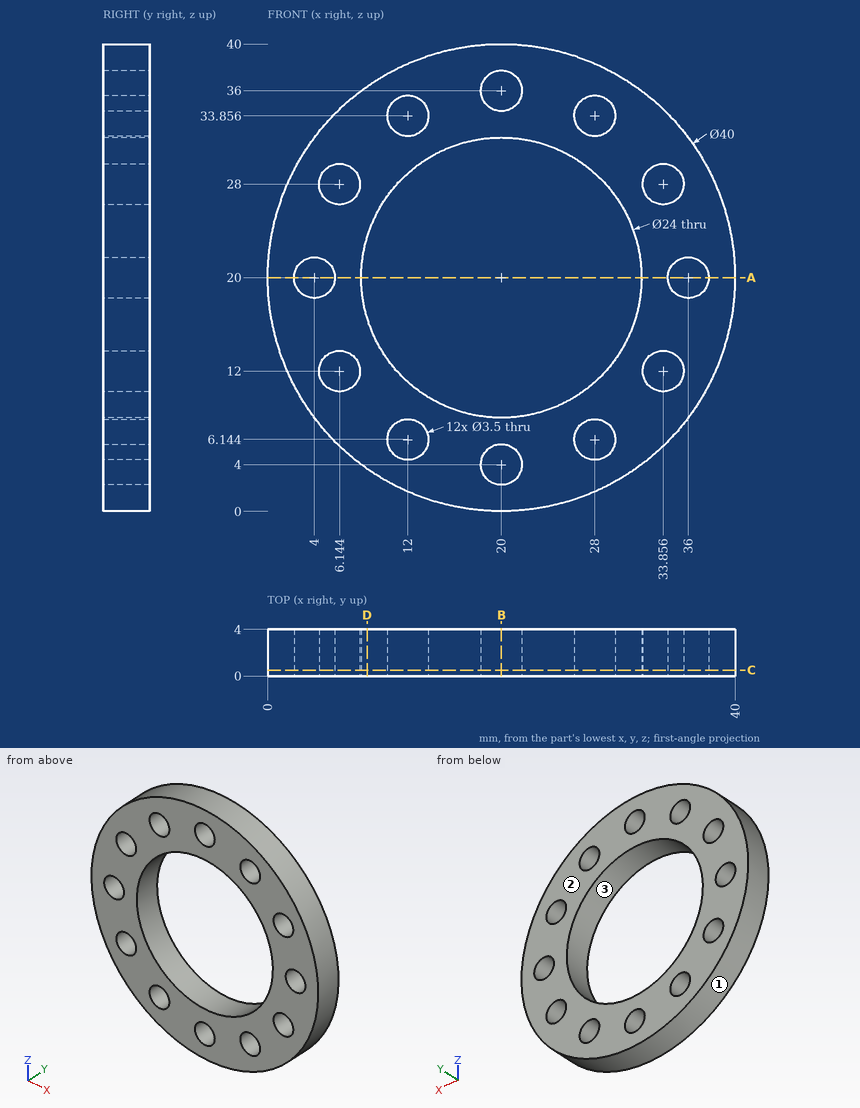
Source: three-view drawing plus pictorial views. Frame: mm from the lowest corner of the part. Give positions to 0.01 mm unless a question says otherwise; leave off trailing zeros. Write each loop counter-clockwise with the first axis right and the second up, starting at its lowest first coordinate (ties: lowest second). Pieces come first, ordered by that corner, then holes. Notation, with made-up numbers: (80, 40) - (90, 40) arc R29 ccw to (90, 74) - close; hole circle Ø7 at (49.5, 81). An arc over 180 degrees is marked (long way). Write item = value, one per line. Start each with the question number.
1. Section query A-A, the plane z = 20. Output: boundary loops of the cut face in (x, y), then the cut area to 3 significant figures.
2. Ray query, L1, parallel to X at y = 2.3, z = 20; L2, parallel to X at y = 0.8, z = 6 (1 decimal); L3, parallel to X at y = 2.95, z = 28 (1 decimal). Return the intervals inside material, ascending.
3. First-contact query: pin 1 Ø1 at (x, y) = (6, 2) entering from -Z (1 decimal); pin 2 Ø4.5 at (x, z) = (12, 6.14) entering from -Y; pin 3 Ø1 at (y, z) = (2.5, 23) entering from +X; pin 4 Ø1.5 at (x, y) = (22.5, 2) entering from -Z. Flat tips, straight axial feed; report the tip coordinate or a pass-through.
4. Section query D-D, the plane x = 8.5. Output: boundary loops of the cut face in (y, z).
5. Section query C-C, the plane y = 0.5. Count the separate pieces of the cut face and the enclosed holes in it, then the cut area to 3 significant figures.
6. Mould query, pull axis Z, two halves, no side actions, for the marked faces 1, 2 and 3. Classes: released by +Z, released by -Z, zero draft, split by the parting line, or undercut.
7. Section query B-B, the plane x = 20. Output: boundary loops of the cut face in (y, z), then the cut area to 3 significant figures.
Check sheet entries:
q1.outline = (0, 0) - (2.25, 0) - (2.25, 4) - (0, 4) - close; (5.75, 0) - (8, 0) - (8, 4) - (5.75, 4) - close; (32, 0) - (34.25, 0) - (34.25, 4) - (32, 4) - close; (37.75, 0) - (40, 0) - (40, 4) - (37.75, 4) - close
q1.area = 36.0 mm2
q2.L1 = 0 to 2.25, 5.75 to 8, 32 to 34.25, 37.75 to 40
q2.L2 = 5.7 to 10.3, 13.7 to 26.3, 29.7 to 34.3
q2.L3 = 1.7 to 4.4, 7.9 to 11.1, 28.9 to 32.1, 35.6 to 38.3
q3.pin_1 = 5.2
q3.pin_2 = 0
q3.pin_3 = 39.84
q3.pin_4 = 0.08
q4.outline = (0, 3.64) - (4, 3.64) - (4, 16.57) - (0, 16.57) - close; (0, 23.43) - (4, 23.43) - (4, 36.36) - (0, 36.36) - close
q5.separate_pieces = 1
q5.enclosed_holes = 13
q5.area = 689 mm2
q6.face_1 = split by the parting line
q6.face_2 = zero draft
q6.face_3 = undercut
q7.outline = (0, 0) - (4, 0) - (4, 2.25) - (0, 2.25) - close; (0, 5.75) - (4, 5.75) - (4, 8) - (0, 8) - close; (0, 32) - (4, 32) - (4, 34.25) - (0, 34.25) - close; (0, 37.75) - (4, 37.75) - (4, 40) - (0, 40) - close
q7.area = 36.0 mm2
